Verification items for the finished model (mm, model axes). Give positions to 0.01 mm unless a question says otherwise; leave off trailing zeros. Loops run counter-clockwise (first coordinate to the right, second up) from the corner with the lowest first, then second, coordinate; pieces in that order, holes last. Notation, with made-up numbers: (69.5, 54.25) - (108.5, 54.25) arc R14 cw to (108.5, 81.25) - close; hole circle Ø11 at (29, 88.25). An arc over 180 degrees is marked (long way). Put each result on its own line as item: value. Start each with the question number.
```python
from build123d import *

# Parameters (mm, degrees)
SKETCH1_R           = 3.175
BOSS_EXTRUDE1_DEPTH = 6.35
SKETCH3_R           = 6.35
CUT_EXTRUDE1_DEPTH  = 6.35
SKETCH4_R           = 2.413
CUT_EXTRUDE2_DEPTH  = 6.35


with BuildPart() as part:
    # Sketch1 → Boss-Extrude1 (new body)
    with BuildSketch(Plane.XY):
        with BuildLine():
            Line((-388.789077681, 181.190585859), (-388.789077681, 143.090585859))
            ThreePointArc((-388.789077681, 143.090585859), (-386.929205741, 138.600457798), (-382.439077681, 136.740585859))
            ThreePointArc((-382.439077681, 136.740585859), (-350.689077681, 139.944338866), (-318.939077681, 136.740585859))
            ThreePointArc((-318.939077681, 136.740585859), (-314.44894962, 138.600457798), (-312.589077681, 143.090585859))
            Line((-312.589077681, 143.090585859), (-312.589077681, 181.190585859))
            ThreePointArc((-312.589077681, 181.190585859), (-314.44894962, 185.680713919), (-318.939077681, 187.540585859))
            ThreePointArc((-318.939077681, 187.540585859), (-350.689077681, 184.336832851), (-382.439077681, 187.540585859))
            ThreePointArc((-382.439077681, 187.540585859), (-386.929205741, 185.680713919), (-388.789077681, 181.190585859))
        make_face()
        with Locations((-382.439077681, 181.190585859)):
            Circle(SKETCH1_R, mode=Mode.SUBTRACT)
        with Locations((-318.939077681, 181.190585859)):
            Circle(SKETCH1_R, mode=Mode.SUBTRACT)
        with Locations((-382.439077681, 143.090585859)):
            Circle(SKETCH1_R, mode=Mode.SUBTRACT)
        with Locations((-318.939077681, 143.090585859)):
            Circle(SKETCH1_R, mode=Mode.SUBTRACT)
    extrude(amount=BOSS_EXTRUDE1_DEPTH)

    # Sketch3 → Cut-Extrude1 (cut)
    with BuildSketch(Plane.XY.offset(6.35)):
        with Locations((-350.689077681, 162.140585859)):
            Circle(SKETCH3_R)
    extrude(amount=-CUT_EXTRUDE1_DEPTH, mode=Mode.SUBTRACT)

    # Sketch4 → Cut-Extrude2 (cut)
    with BuildSketch(Plane.XY.offset(6.35)):
        with Locations((-337.989077681, 171.665585859)):
            Circle(SKETCH4_R)
        with Locations((-337.989077681, 152.615585859)):
            Circle(SKETCH4_R)
        with Locations((-363.389077681, 152.615585859)):
            Circle(SKETCH4_R)
        with Locations((-363.389077681, 171.665585859)):
            Circle(SKETCH4_R)
    extrude(amount=-CUT_EXTRUDE2_DEPTH, mode=Mode.SUBTRACT)


solid = part.part
```
1) Section check D-D, the plane x = -339. Enter the section's corners in (y, z), plus the area to 3 significant figures.
2) Section check B-B, the plane y = 164. Enter the section's corners in (x, z), plus the area to 3 significant figures.
3) Draft check along Y on faces 1 (the face through (-386.88, 185.73, 3.13)), 2 (the face through (-351.137, 139.944, 3.131)), 3 (the face through (-388.789, 162, 3)), 4 (the face through (-316.01, 179.97, 3.13)). Enter one of: pulls with the +Y half, pulls with the -Y half, needs draft (parallel to the pull), parting line crosses it, or undercut.
4) Scan lines: line 1 along Y through (x, z) = (-384, 1.5); line 2 along X through (y, z) = (144, 1.75); line 3 along Y through (x, z) = (-317, 6.25). Record each from-to range of solid material in increasing order. Write a range as from..to.
5) Section check C-C, the plane z = 1.75. State how many separate pieces and enclosed holes the cut face has, plus the area to 3 significant figures.
6) Section check A-A, the plane x = -354. Enter the section's corners in (y, z), plus the area to 3 significant figures.
7) Depth check by flat-ended pin: P1, Ø5.5, axis at x = -318.94, y = 143.09, coming from the +Z side; P2, Ø1.5, axis at x = -321.5, z = 5, coming from the +Y side; P3, Ø1.5, axis at x = -338, z = 4, coming from the +Y side. Enter the tip coordinate at first touch or a pass-through.
Results are:
1. outline: (139.51, 0) - (150.42, 0) - (150.42, 6.35) - (139.51, 6.35) - close; (154.81, 0) - (169.47, 0) - (169.47, 6.35) - (154.81, 6.35) - close; (173.86, 0) - (184.77, 0) - (184.77, 6.35) - (173.86, 6.35) - close
1. area: 232 mm2
2. outline: (-388.79, 0) - (-356.76, 0) - (-356.76, 6.35) - (-388.79, 6.35) - close; (-344.62, 0) - (-312.59, 0) - (-312.59, 6.35) - (-344.62, 6.35) - close
2. area: 407 mm2
3. face 1: pulls with the +Y half
3. face 2: pulls with the -Y half
3. face 3: needs draft
3. face 4: undercut
4. line 1: y = 136.94..140.33, 145.86..178.43, 183.96..187.35
4. line 2: x = -388.79..-385.48, -379.4..-321.98, -315.9..-312.59
4. line 3: y = 137.04..140.58, 145.6..178.68, 183.7..187.24
5. separate pieces: 1
5. enclosed holes: 9
5. area: 3,240 mm2
6. outline: (139.91, 0) - (156.72, 0) - (156.72, 6.35) - (139.91, 6.35) - close; (167.56, 0) - (184.37, 0) - (184.37, 6.35) - (167.56, 6.35) - close
6. area: 214 mm2
7. P1: passes through
7. P2: stops at y = 187.18
7. P3: stops at y = 184.91
